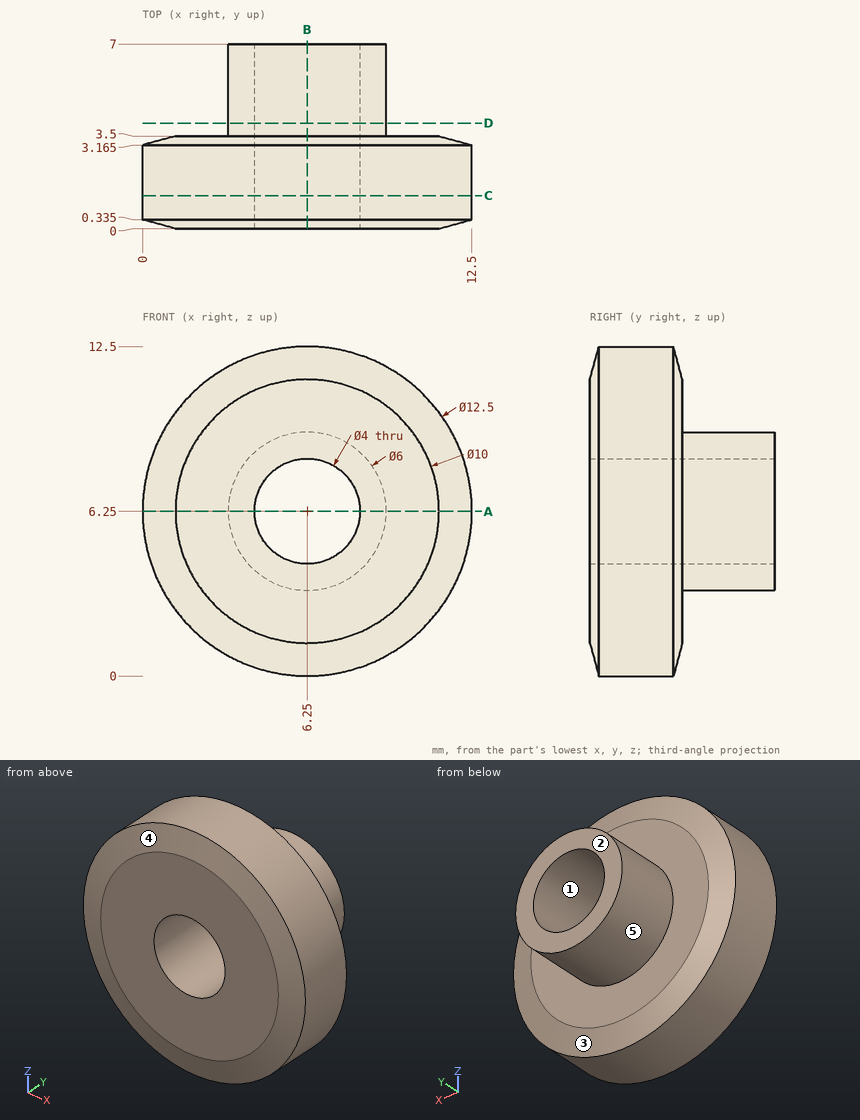
Print and shaded views of the part. All mm, measured from the part's lowest x, y and z. A direction names the side the tool comes from. Coordinates: 2 decimals unless noted, no trailing zeros. Order: outer loops, then holes, each group sorted by start corner. A loop starts at its lowest first (then second) coordinate and runs counter-clockwise, first axis right, second up. Notation, with made-up numbers: M 76,-10 L 89,-10 A31 cw 89,29 Z; hole C -11,67.25 d5. An arc over 180 degrees is marked long. Write each question's results on one line, items separated by ' | '. Start each with the question number.
Q1. Cut at A-A (z = 6.25). List the corners of the cut face in (x, y) (3 decimals), then the cut area to 3 significant figures.
Q2. Cut at D-D (y = 4). List the corners of the cut face in (x, z).
Q3. Flat gauge pins, fed straight in: P1, Ø2.5, axis at x = 6.25, z = 6.25, coming from the +Y side; P2, Ø1.5, axis at x = 1.5, z = 6.5, coming from the +Y side; P3, Ø2, axis at y = 2, z = 10, coming from the +X side; P4, Ø1, axis at y = 5.5, z = 5.5, coming from the -X side. Where does each tip first touch, or does it go through?
Q4. Cut at C-C (y = 1.25). List the corners of the cut face in (x, z), then the cut area to 3 significant figures.
Q5. Which spindle directions (+Z, -Z, +X, -X, +Y, -Y) get a long thin tool onto all of the face, cutting with end or side? Do the marked faces 4 and 5. Say none if no direction does.
Q6. Pull direction Z, two halves, no side cores. Call the marked faces 1, 2 and 3: +Z half, -Z half, draft (parallel to the pull), parting line (faces both ways), or undercut.
Q7. Drill centre lines: probe 1 along Z at (x, y) = (6.25, 5.25); probe 2 along Z at (x, y) = (6.25, 1.75); probe 3 along Y at (x, z) = (5.25, 2.25). Where is each one in solid material? Low to high. Write a range as from..to.
Q8. Cut at B-B (x = 6.25). List the corners of the cut face in (y, z) (3 decimals).
Found:
1) outline: M 0,0.335 L 1.25,0 L 4.25,0 L 4.25,7 L 3.25,7 L 3.25,3.5 L 1.25,3.5 L 0,3.165 Z; M 8.25,0 L 11.25,0 L 12.5,0.335 L 12.5,3.165 L 11.25,3.5 L 9.25,3.5 L 9.25,7 L 8.25,7 Z | area: 35.9 mm²
2) outline: C 6.25,6.25 d6; hole C 6.25,6.25 d4
3) P1: through | P2: y = 3.5 | P3: x = 11.86 | P4: x = 3.26
4) outline: C 6.25,6.25 d12.5; hole C 6.25,6.25 d4 | area: 110 mm²
5) face 4: -Y | face 5: +Y
6) face 1: undercut | face 2: draft | face 3: parting line
7) probe 1: 3.25..4.25, 8.25..9.25 | probe 2: 0..4.25, 8.25..12.5 | probe 3: 0..3.5
8) outline: M 0,1.25 L 0.335,0 L 3.165,0 L 3.5,1.25 L 3.5,3.25 L 7,3.25 L 7,4.25 L 0,4.25 Z; M 0,8.25 L 7,8.25 L 7,9.25 L 3.5,9.25 L 3.5,11.25 L 3.165,12.5 L 0.335,12.5 L 0,11.25 Z
